Could you check a few things on this model? Use its own coordinates, in mm. Coordinates: 2 decimals unless noted, no trailing zeros. Write each loop counter-clockwise with the first axis right and the second up, starting at its lowest first coordinate (ties: lowest second). Pieces come first, ordered by that corner, then holes.
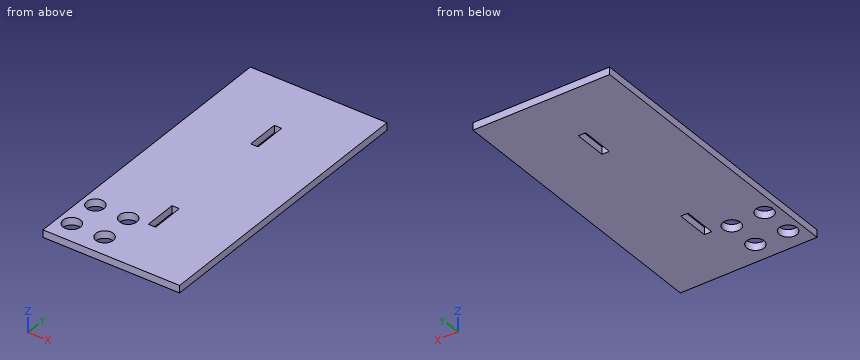
Autodesk Inventor part; units mm, degrees
ref_plane "YZ Plane" through (0, 0, 0) normal (1, 0, 0) x (0, 1, 0)
ref_plane "XZ Plane" through (0, 0, 0) normal (0, 1, 0) x (-1, 0, 0)
ref_plane "XY Plane" through (0, 0, 0) normal (0, 0, 1) x (1, 0, 0)
sketch "Sketch1" plane through (0, 0, 0) normal (0, 0, 1) x (1, 0, 0)
  line L0 (0, 0) -> (125, 0)
  line L1 (125, 0) -> (125, 263.462)
  line L2 (125, 263.462) -> (0, 263.462)
  line L3 (0, 263.462) -> (0, 0)
  dimension "d0" = 263.462
  dimension "d1" = 125
extrude "Extrusion1" add sketch "Sketch1" along normal blind 6.731
sketch "Sketch2" plane through (0, 0, 6.731) normal (0, 0, 1) x (1, 0, 0)
  line L0 (125, 263.462) -> (0, 263.462)
  line L1 (0, 263.462) -> (0, 0)
  line L2 (59.1345, 211.731) -> (65.8655, 211.731)
  line L3 (65.8655, 211.731) -> (65.8655, 181.731)
  line L4 (65.8655, 181.731) -> (59.1345, 181.731)
  line L5 (59.1345, 181.731) -> (59.1345, 211.731)
  line L6 (59.1345, 81.731) -> (65.8655, 81.731)
  line L7 (65.8655, 81.731) -> (65.8655, 51.731)
  line L8 (65.8655, 51.731) -> (59.1345, 51.731)
  line L9 (59.1345, 51.731) -> (59.1345, 81.731)
  line L10 (62.5, 81.731) -> (62.5, 181.731) construction
  point P0 (62.5, 131.731)
  point P1 (0, 131.731)
  point P2 (62.5, 263.462)
  dimension "d4" = 30
  dimension "d5" = 100
  dimension "d6" = 6.731
extrude "Extrusion2" cut sketch "Sketch2" against normal up to next
sketch "Sketch3" plane through (0, 0, 6.731) normal (0, 0, 1) x (1, 0, 0)
  line L0 (0, 263.462) -> (0, 0)
  line L1 (12.5, 19.231) -> (12.5, 49.231) construction
  line L2 (12.5, 49.231) -> (42.5, 49.231) construction
  line L3 (0, 0) -> (125, 0)
  point P0 (42.5, 19.231)
  dimension "d9" = 30
  dimension "d10" = 12.5
  dimension "d18" = 19.231
hole "Hole1" at (12.5, 49.231, 6.731) at (42.5, 49.231, 6.731) at (42.5, 19.231, 6.731) at (12.5, 19.231, 6.731) direction (0, 0, -1) diameter 16 end through all
equation "\"d2\" = THICKB"
equation "\"d6\" = THICKB"
equation "\"d7\" = THICKB"
equation "\"d18\" = THICKB + d10"
equation "\"THICKA\" = 3.175"
equation "\"THICKB\" = 6.731"
equation "\"THICKC\" = 12.7"
equation "\"THICKPLY\" = 5"
equation "\"MAGDIA\" = 9.5"
equation "\"BALLDIA\" = 12"
properties part number "Top"
Item 1: If I drill on line 1 along Y through (x, z) = (12.5, 1.75); line 2 along X through (y, z) = (77.5, 1); line 3 along X through (y, z) = (53, 6.5), over which ranges is the centre line in solid material (lowest first)?
Item 2: I want a section at A-A, the plane z = 2.5. List the corners of the cut face in (x, y) for me, then the cut area to 3 significant figures.
Item 3: I want a section at B-B, the plane x = 42.5. List the corners of the cut face in (y, z) for me.
Taken from the geometry:
1. line 1: y = 0 to 11.23, 27.23 to 41.23, 57.23 to 263.46
1. line 2: x = 0 to 59.13, 65.87 to 125
1. line 3: x = 0 to 5.44, 19.56 to 35.44, 49.56 to 59.13, 65.87 to 125
2. outline: (0, 0) - (125, 0) - (125, 263.46) - (0, 263.46) - close; hole circle Ø16 at (12.5, 19.23); hole circle Ø16 at (12.5, 49.23); hole circle Ø16 at (42.5, 19.23); hole circle Ø16 at (42.5, 49.23); hole (59.13, 51.73) - (65.87, 51.73) - (65.87, 81.73) - (59.13, 81.73) - close; hole (59.13, 181.73) - (65.87, 181.73) - (65.87, 211.73) - (59.13, 211.73) - close
2. area: 31,700 mm2
3. outline: (0, 0) - (11.23, 0) - (11.23, 6.73) - (0, 6.73) - close; (27.23, 0) - (41.23, 0) - (41.23, 6.73) - (27.23, 6.73) - close; (57.23, 0) - (263.46, 0) - (263.46, 6.73) - (57.23, 6.73) - close
